from build123d import *

# Parameters (mm, degrees)
SKETCH1_R           = 4.2
BOSS_EXTRUDE1_DEPTH = 5
SKETCH2_R           = 4.2
BOSS_EXTRUDE2_DEPTH = 1


with BuildPart() as part:
    # Sketch1 → Boss-Extrude1 (new body)
    with BuildSketch(Plane(origin=(0, 0, 0), x_dir=(1, 0, 0), z_dir=(0, 1, 0))):
        with BuildLine():
            ThreePointArc((2.070552361, 7.72740661), (0, 10.088419076), (-2.070552361, 7.72740661))
            ThreePointArc((-2.070552361, 7.72740661), (-2.955790462, 5.119579257), (-5.656854249, 5.656854249))
            ThreePointArc((-5.656854249, 5.656854249), (-8.736827203, 5.044209538), (-7.72740661, 2.070552361))
            ThreePointArc((-7.72740661, 2.070552361), (-5.911580924, 0), (-7.72740661, -2.070552361))
            ThreePointArc((-7.72740661, -2.070552361), (-8.736827203, -5.044209538), (-5.656854249, -5.656854249))
            ThreePointArc((-5.656854249, -5.656854249), (-2.955790462, -5.119579257), (-2.070552361, -7.72740661))
            ThreePointArc((-2.070552361, -7.72740661), (0, -10.088419076), (2.070552361, -7.72740661))
            ThreePointArc((2.070552361, -7.72740661), (2.955790462, -5.119579257), (5.656854249, -5.656854249))
            ThreePointArc((5.656854249, -5.656854249), (8.736827203, -5.044209538), (7.72740661, -2.070552361))
            ThreePointArc((7.72740661, -2.070552361), (5.911580924, 0), (7.72740661, 2.070552361))
            ThreePointArc((7.72740661, 2.070552361), (8.736827203, 5.044209538), (5.656854249, 5.656854249))
            ThreePointArc((5.656854249, 5.656854249), (2.955790462, 5.119579257), (2.070552361, 7.72740661))
        make_face()
        with Locations(Location((0, 0, 0), (0, 0, 270))):
            Circle(SKETCH1_R, mode=Mode.SUBTRACT)
    extrude(amount=BOSS_EXTRUDE1_DEPTH)

    # Sketch2 → Boss-Extrude2 (add)
    with BuildSketch(Plane.XZ):
        with Locations(Location((0, 0, 0), (0, 0, 270))):
            Circle(SKETCH2_R)
        Polygon((0, 2.424871131), (-2.1, 1.212435565), (-2.1, -1.212435565), (0, -2.424871131), (2.1, -1.212435565), (2.1, 1.212435565), align=None, mode=Mode.SUBTRACT)
    extrude(amount=-BOSS_EXTRUDE2_DEPTH)


solid = part.part
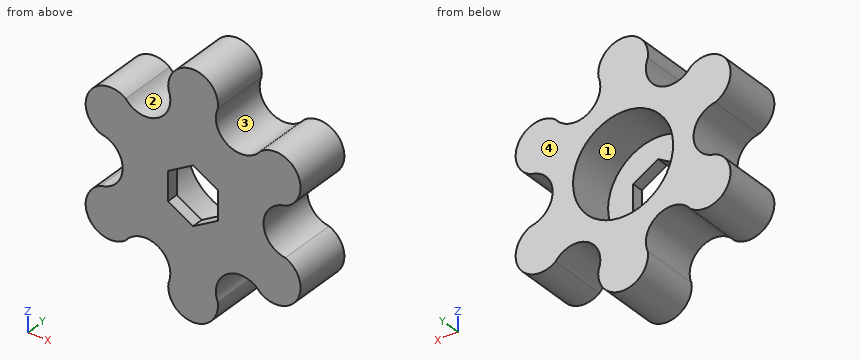
Work out the finished part from the listing and answer in its coordinate system (mm). Face numbers are marked on the shaded views. A direction names the side the tool comes from. Round coordinates to 2 decimals unless told otherwise and drop trailing zeros. Write each loop counter-clockwise with the first axis right and the second up, starting at its lowest first coordinate (ties: lowest second). Pieces come first, ordered by that corner, then holes. Notation, with made-up numbers: (76, 1) - (126, 1) arc R30 ccw to (126, 32) - close; hole circle Ø11 at (-28, -36). An arc over 180 degrees is marked (long way). Answer in a Markdown table with one row per item. Add a question column.
1. Find the intervals of material crossed by line 1 along X through (y, z) = (2.45, 5.25); line 2 along Z through (x, y) = (7.75, 3.45); line 3 along Y through (x, z) = (1.75, 2), in increasing order. Write a range as from..to.
2. For the marked faces 1 and 2, determine the directions among +Z, -Z, +X, -X, +Y, -Y from which every point of the face is accessible in a straight line to the end or side of a thin tool.
3. A cutting plane is placed at C-C, the plane z = 8. Determine the outline of the cut face in (x, y), and give its area (3 significant figures).
4. A cutting plane is placed at A-A, the plane x = -1. Determine the outline of the cut face in (y, z), and give its area (3 significant figures).
5. The mould has two halves that part along Z. Classify the marked faces 3 and 4: +Z half, -Z half, draft (parallel to the pull), parting line (faces both ways), or undercut.
6. Given pin 1 (10 mm diameter, centred on x = -4.5, z = -3.5, fed in from -Y); pin 2 (0.8 mm diameter, centred on y = 0.5, z = -0.5, fed in from -X); pin 3 (0.8 mm diameter, centred on y = 0.5, z = -0.5, fed in from +X); pin 4 (1 mm diameter, centred on x = -7, y = 1, fed in from -Z), each flat-ended and moving along its own axis, determine where each tip first touches the part or whether it passes through.
7. A cutting plane is placed at B-B, the plane y = 4.15. Determine the outline of the cut face in (x, z).
8. A cutting plane is placed at D-D, the plane x = 2.75. Determine the outline of the cut face in (y, z).
Worked out:
| question | item | result |
|---|---|---|
| 1 | line 1 | -8.6..-5.24, -2.76..2.76, 5.24..8.6 |
| 1 | line 2 | -5.92..-2.08, 2.08..5.92 |
| 1 | line 3 | 0..1 |
| 2 | face 1 | +Y |
| 2 | face 2 | +Y, -Y |
| 3 | outline | (-2.09, 0) - (2.09, 0) - (2.09, 5) - (-2.09, 5) - close |
| 3 | area | 20.9 mm^2 |
| 4 | outline | (0, -9.83) - (5, -9.83) - (5, -4.08) - (1, -4.08) - (1, -1.85) - (0, -1.85) - close; (0, 1.85) - (1, 1.85) - (1, 4.08) - (5, 4.08) - (5, 9.83) - (0, 9.83) - close |
| 4 | area | 62.0 mm^2 |
| 5 | face 3 | undercut |
| 5 | face 4 | draft |
| 6 | pin 1 | y = 0 |
| 6 | pin 2 | x = -6.12 |
| 6 | pin 3 | x = 6.12 |
| 6 | pin 4 | z = -6.09 |
| 7 | outline | (-7.73, -2.07) arc R2.09 ccw (long way) to (-5.66, -5.66) arc R2.09 cw to (-2.07, -7.73) arc R2.09 ccw (long way) to (2.07, -7.73) arc R2.09 cw to (5.66, -5.66) arc R2.09 ccw (long way) to (7.73, -2.07) arc R2.09 cw to (7.73, 2.07) arc R2.09 ccw (long way) to (5.66, 5.66) arc R2.09 cw to (2.07, 7.73) arc R2.09 ccw (long way) to (-2.07, 7.73) arc R2.09 cw to (-5.66, 5.66) arc R2.09 ccw (long way) to (-7.73, 2.07) arc R2.09 cw to start; hole circle Ø8.4 at (0, 0) |
| 8 | outline | (0, -5.26) - (5, -5.26) - (5, -3.17) - (1, -3.17) - (1, 3.17) - (5, 3.17) - (5, 5.26) - (0, 5.26) - close |
